Answer from the drawing. Dimensions are ordinates in mm from the lowest x, y and z of the part. A direction names the side the tool comes from. Coordinates: 2 decimals unless noted, no trailing zeros. Order: outer loops, then holes, each group sorted by start corner. A loop starts at its lowest first (then second) coordinate and runs counter-clockwise, first axis right, second up. Notation, with made-up numbers: M -14,30.25 L 0,30.25 A25 ccw 0,54.25 Z; hole C 66,-2.5 d6. An arc over 180 degrees is marked long. Use a Markdown table: item, result.
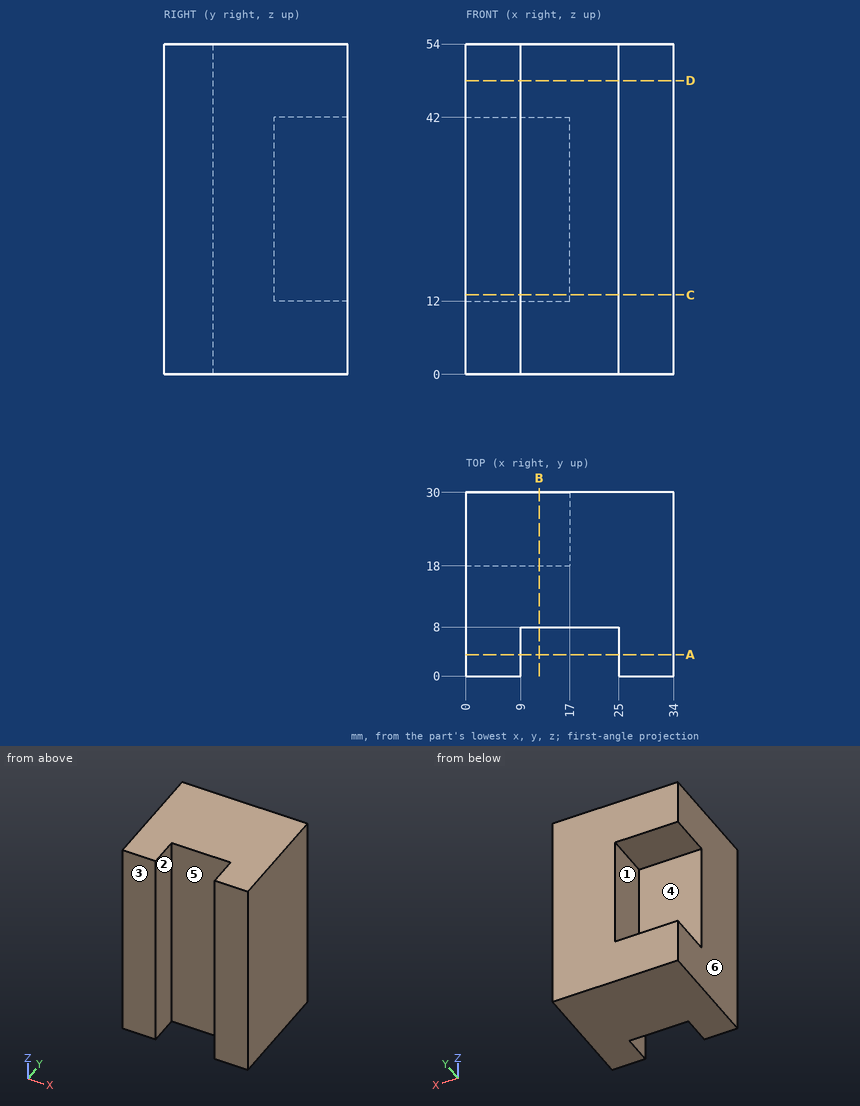
(1) Which of the six approach directions +Z, -Z, +X, -X, +Y, -Y give full straight-line access (tool end or side, diameter ignored) to the marked faces 1, 2 and 3?
Conclusion:
| item | result |
|---|---|
| face 1 | -X, +Y |
| face 2 | +Z, -Z, -Y |
| face 3 | +Z, -Z, +X, -X, -Y |
(2) Determine the mould class of the marked faces 4, 5 and 6 for opening direction X: pulls with the +X half, pulls with the -X half, needs draft (parallel to the pull), parting line crosses it, or undercut.
Conclusion:
| item | result |
|---|---|
| face 4 | needs draft |
| face 5 | undercut |
| face 6 | pulls with the -X half |
(3) A cutting plane is placed at B-B (x = 12). Determine the outline of the cut face in (y, z).
Conclusion:
| item | result |
|---|---|
| outline | M 8,0 L 30,0 L 30,12 L 18,12 L 18,42 L 30,42 L 30,54 L 8,54 Z |
(4) A cutting plane is placed at D-D (z = 48). Determine the outline of the cut face in (x, y).
Conclusion:
| item | result |
|---|---|
| outline | M 0,0 L 9,0 L 9,8 L 25,8 L 25,0 L 34,0 L 34,30 L 0,30 Z |
(5) Straight lines are drawn through the part: L1, parallel to Z at x = 9.5, y = 21; L2, parallel to Y at x = 4, z = 41.5; L3, parallel to X at y = 18.25, z = 12.5. For each, find the intervals that lie inside material, in ascending order.
Conclusion:
| item | result |
|---|---|
| L1 | 0 to 12, 42 to 54 |
| L2 | 0 to 18 |
| L3 | 17 to 34 |
(6) A cutting plane is placed at C-C (z = 13). Determine the outline of the cut face in (x, y).
Conclusion:
| item | result |
|---|---|
| outline | M 0,0 L 9,0 L 9,8 L 25,8 L 25,0 L 34,0 L 34,30 L 17,30 L 17,18 L 0,18 Z |
(7) A cutting plane is placed at A-A (y = 3.5). Determine the outline of the cut face in (x, z).
Conclusion:
| item | result |
|---|---|
| outline | M 0,0 L 9,0 L 9,54 L 0,54 Z; M 25,0 L 34,0 L 34,54 L 25,54 Z |
(8) Given P1, Ø6.5, axis at y = 6, z = 31, coming from the -X side; P2, Ø5, axis at x = 7.5, z = 23.5, coming from the +Y side; P3, Ø6, axis at x = 19.5, z = 18.5, coming from the -Y side, each flat-ended and moving along its own axis, determine where each tip first touches the part or whether it passes through.
Conclusion:
| item | result |
|---|---|
| P1 | x = 0 |
| P2 | y = 18 |
| P3 | y = 8 |
